Geometry check sheet. Reference: the model listing, model coordinates, mm. Face numbers are marked on the shaded views. Give positions to 0.01 mm unless a question says otherwise; leave off trailing zeros. Loops run counter-clockwise (first coordinate to the right, second up) from the corner with the lowest first, then second, coordinate; pieces in that order, holes last. Notation, with made-up numbers: (86.5, 30) -> (136.5, 30) arc R26 cw to (136.5, 45) -> close; hole circle Ø8 at (-30.5, 14.25). An arc over 180 degrees is marked (long way). Answer as a JSON object with one key per item and string values.
from build123d import *

# Parameters (mm, degrees)
SKETCH1_R           = 5
BOSS_EXTRUDE1_DEPTH = 25
SKETCH2_R           = 10
BOSS_EXTRUDE2_DEPTH = 5
FILLET1_R           = 7.5


with BuildPart() as part:
    # Sketch1 → Boss-Extrude1 (new, symmetric)
    with BuildSketch(Plane.XY):
        Circle(SKETCH1_R)
    extrude(amount=BOSS_EXTRUDE1_DEPTH, both=True)

    # Sketch2 → Boss-Extrude2 (add)
    with BuildSketch(Plane.XY.offset(25)):
        Circle(SKETCH2_R)
    boss_extrude2 = extrude(amount=BOSS_EXTRUDE2_DEPTH)

    # Mirror1: Boss-Extrude2 across plane
    add(boss_extrude2.mirror(Plane.XY))

    # Fillet1
    # the kernel refuses this fillet: 7.5 mm, written as the material it takes off along each edge
    with BuildSketch(Plane(origin=(0, 0, 30), x_dir=(1, 0, 0), z_dir=(0, -1, 0))) as fillet1_piece_1:
        with BuildLine():
            CenterArc((2.928932188, -7.5), FILLET1_R, 19.471220634, 70.528779366)
            Line((2.928932188, 0), (2.928932188, 0.15))
            Line((2.928932188, 0.15), (10, 0.15))
            Line((10, 0.15), (10.15, 0))
            ThreePointArc((10.15, 0), (10.15, -2.5), (10.141421356, -4.95))
            Line((10.141421356, -4.95), (10, -5))
        make_face()
    revolve(axis=Axis((0, 0, 30), (0, 0, 1)), mode=Mode.SUBTRACT)


solid = part.part
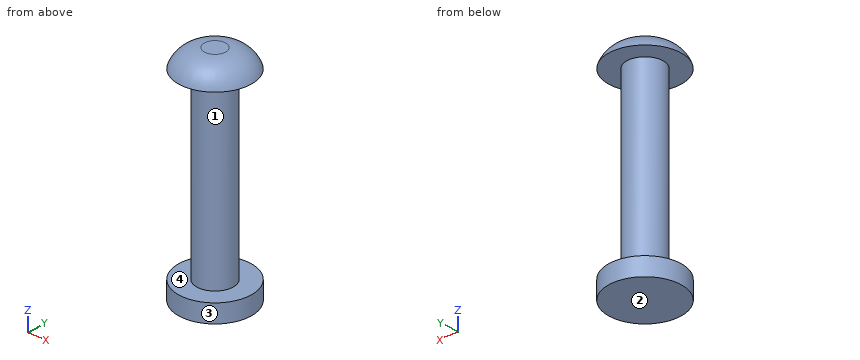
1) Section check A-A on z = 18. Record the cut outline in (x, y).
Geometry check:
{"outline": "circle Ø10 at (0, 0)"}
2) Draft check along Z on the marked faces 1, 2, 3 and 4. Enter one of: pulls with the +Z half, pulls with the -Z half, needs draft (parallel to the pull), parting line crosses it, or undercut.
Geometry check:
{"face 1": "undercut", "face 2": "pulls with the -Z half", "face 3": "needs draft", "face 4": "undercut"}
3) Material ranges on line 1 along Z through (x, y) = (5.25, -7.25); line 2 along Z through (x, y) = (-1, -5.75); line 3 along Y through (x, z) = (-3.75, -10.5), recorded low to high. Write a range as from..to.
Geometry check:
{"line 1": "z = -30..-25, 25..26.97", "line 2": "z = -30..-25, 25..29.41", "line 3": "y = -3.31..3.31"}
4) Depth check by flat-ended pin: P1, Ø4, axis at x = -6, z = 8.5, coming from the +Y side; P2, Ø12, axis at y = -1, z = 2.5, coming from the -X side; P3, Ø8, axis at x = -1, y = 7, coming from the +Z side. Enter the tip coordinate at first touch or a pass-through.
Geometry check:
{"P1": "stops at y = 3", "P2": "stops at x = -5", "P3": "stops at z = 30"}
